```python
from build123d import *

# Parameters (mm, degrees)
SKETCH_1_R               = 20
EXTRUDE_1_DEPTH          = 12
SKETCH_3_R               = 34
EXTRUDE_2_DEPTH          = 12
SKETCH_4_R               = 22
EXTRUDE_3_DEPTH          = 42
SKETCH_5_R               = 17.5
EXTRUDE_5_DEPTH          = 39
SKETCH_6_R               = 12.5
EXTRUDE_6_DEPTH          = 12
SKETCH_8_R               = 16
SKETCH_8_R_2             = 10
EXTRUDE_7_DEPTH          = 18
SKETCH_11_R              = 3
CUT_EXTRUDE_9_DEPTH      = 12
PATTERN_CIRCULAR_1_COUNT = 4
SKETCH_12_R              = 14
EXTRUDE_8_DEPTH          = 17
SKETCH_14_R              = 5
CUT_EXTRUDE_10_DEPTH     = 15


with BuildPart() as part:
    # 草图1 → 凸台-拉伸1 (new body)
    with BuildSketch(Plane(origin=(0, 0, 0), x_dir=(1, 0, 0), z_dir=(0, 1, 0))):
        with Locations(Location((0, 0, 0), (0, 0, 270))):
            Circle(SKETCH_1_R)
    extrude(amount=EXTRUDE_1_DEPTH)

    # 草图3 → 凸台-拉伸2 (add)
    with BuildSketch(Plane.XZ):
        with Locations(Location((0, 0, 0), (0, 0, 270))):
            Circle(SKETCH_3_R)
    extrude(amount=EXTRUDE_2_DEPTH)

    # 草图4 → 凸台-拉伸3 (add)
    with BuildSketch(Plane.XZ.offset(12)):
        with Locations(Location((0, 0, 0), (0, 0, 90))):
            Circle(SKETCH_4_R)
    extrude(amount=EXTRUDE_3_DEPTH)

    # 草图5 → 凸台-拉伸5 (add)
    with BuildSketch(Plane.XZ.offset(54)):
        with Locations(Location((0, 0, 0), (0, 0, 270))):
            Circle(SKETCH_5_R)
    extrude(amount=EXTRUDE_5_DEPTH)

    # 草图6 → 凸台-拉伸6 (add)
    with BuildSketch(Plane.XZ.offset(93)):
        with Locations(Location((0, 0, 0), (0, 0, 270))):
            Circle(SKETCH_6_R)
    extrude(amount=EXTRUDE_6_DEPTH)

    # 草图8 → 凸台-拉伸7 (add)
    with BuildSketch(Plane.XZ.offset(12)):
        Circle(SKETCH_8_R)
        Circle(SKETCH_8_R_2, mode=Mode.SUBTRACT)
    extrude(amount=EXTRUDE_7_DEPTH)

    # 草图11 → 切除-拉伸9 (cut)
    with BuildSketch(Plane.XZ.offset(12)):
        with Locations(Location((0, 28, 0), (0, 0, 270))):
            Circle(SKETCH_11_R)
    cut_extrude_9 = extrude(amount=-CUT_EXTRUDE_9_DEPTH, mode=Mode.SUBTRACT)

    # 阵列(圆周)1: 切除-拉伸9 ×4 about axis
    pattern_circular_1_axis = Axis((0, 0, 0), (0, 1, 0))
    for i in range(1, PATTERN_CIRCULAR_1_COUNT):
        add(cut_extrude_9.rotate(pattern_circular_1_axis, i * 360 / PATTERN_CIRCULAR_1_COUNT), mode=Mode.SUBTRACT)

    # 草图12 → 凸台-拉伸8 (add)
    with BuildSketch(Plane(origin=(0, 12, 0), x_dir=(1, 0, 0), z_dir=(0, 1, 0))):
        with Locations(Location((0, 0, 0), (0, 0, 270))):
            Circle(SKETCH_12_R)
    extrude(amount=EXTRUDE_8_DEPTH)

    # 草图14 → 切除-拉伸10 (cut)
    with BuildSketch(Plane(origin=(0, 29, 0), x_dir=(1, 0, 0), z_dir=(0, 1, 0))):
        with Locations(Location((0, 0, 0), (0, 0, 270))):
            Circle(SKETCH_14_R)
    extrude(amount=-CUT_EXTRUDE_10_DEPTH, mode=Mode.SUBTRACT)


solid = part.part
```
Can you work these out from the model? Positions are in its coordinate system, mm. A direction names the side the tool comes from. Round coordinates to 2 decimals unless told otherwise and drop trailing zeros. Loops run counter-clockwise (first coordinate to the right, second up) from the corner with the lowest first, then second, coordinate; pieces in that order, holes last. Notation, with made-up numbers: M 77.5,5 L 104.5,5 A34 ccw 104.5,44 Z; hole C 59,-37 d4. An arc over 180 degrees is marked long. Write item = value, one per line. Start each with the question number.
(1) Which directions (+Z, -Z, +X, -X, +Y, -Y) give clear straight access to the entire face, cutting with the end or side of a thin tool? Please do faces 1 (the face through (-19.524, 5.916, -4.336)), 2 (the face through (-10.648, -73.227, 13.887)), 3 (the face through (-31, -6, 0)).
(2) Suppose I cut it at C-C on z = 0. Give the number of separate pieces and of enclosed holes in the cut face, plus the area to 3 significant figures.
(3) I need wall thicknesses on line 1 along X through (y, z) = (-0.5, -2.5); line 2 along Y through (x, z) = (-29.5, -11); line 3 along Y through (x, z) = (16, 1). Which ranges of each line are inside material? Lowest first, please.
(4) If we mould it in two halves opening along X, with no side actions, what happens to faces 4 (the face through (0, 14, 0)), 5 (the face through (10, -54, -15)), 6 (the face through (21.477, -32.706, -4.769))? For each: released by +X, released by -X, zero draft, split by the parting line, or undercut.
(5) Suppose I cut it at B-B on x = -29. Write out the boundary of the cut face in (y, z), plus the area to 3 significant figures.
(6) Suppose I cut it at A-A on z = -28. Write out the boundary of the cut face in (x, y), plus the area to 3 significant figures.
(7) I'm going to push flat-ended pins straight in: P1, Ø8, axis at y = -5, z = -15, coming from the -X side; P2, Ø6, axis at x = 1.5, y = -60.5, coming from the +Z side; P3, Ø9.5, axis at x = 0, z = -28, coming from the +Y side; P4, Ø5, axis at x = 0, z = 28, coming from the +Y side. Where does each tip first touch, or does it pass through?
(8) Suppose I cut it at D-D on x = -16. Write out the boundary of the cut face in (y, z).
Answer block:
q1.face_1 = +Y
q1.face_2 = -Y
q1.face_3 = +Y, -Y
q2.separate_pieces = 3
q2.enclosed_holes = 0
q2.area = 4,990 mm²
q3.line_1 = -33.91 to -29.66, -26.34 to 26.34, 29.66 to 33.91
q3.line_2 = -12 to 0
q3.line_3 = -93 to 12
q4.face_4 = undercut
q4.face_5 = zero draft
q4.face_6 = split by the parting line
q5.outline = M -12,-17.75 L 0,-17.75 L 0,-2.83 L -12,-2.83 Z; M -12,2.83 L 0,2.83 L 0,17.75 L -12,17.75 Z
q5.area = 358 mm²
q6.outline = M -19.29,-12 L -3,-12 L -3,0 L -19.29,0 Z; M 3,-12 L 19.29,-12 L 19.29,0 L 3,0 Z
q6.area = 391 mm²
q7.P1 = -32.17
q7.P2 = 17.5
q7.P3 = 0
q7.P4 = through
q8.outline = M -93,-7.09 L -54,-7.09 L -54,-15.1 L -12,-15.1 L -12,-30 L 0,-30 L 0,-12 L 12,-12 L 12,12 L 0,12 L 0,30 L -12,30 L -12,15.1 L -54,15.1 L -54,7.09 L -93,7.09 Z
